Autodesk Inventor part; units mm, degrees
ref_plane "YZ Plane" through (0, 0, 0) normal (1, 0, 0) x (0, 1, 0)
ref_plane "XZ Plane" through (0, 0, 0) normal (0, 1, 0) x (-1, 0, 0)
ref_plane "XY Plane" through (0, 0, 0) normal (0, 0, 1) x (1, 0, 0)
sketch "Sketch1" plane through (0, 0, 0) normal (0, 0, 1) x (1, 0, 0)
  circle A0 centre (0, 0) radius 22.4676
  circle A1 centre (0, 0) radius 6.35
  point P0 (0, 17.5006)
  point P1 (-17.5006, 0)
  point P2 (0, -17.5006)
  point P3 (17.5006, 0)
  dimension "d0" = 44.9351
  dimension "d1" = 12.7
  dimension "d6" = 35.0012
  dimension "d7" = 17.5006
  dimension "d8" = 17.5006
  dimension "d9" = 17.5006
  dimension "d10" = 17.5006
extrude "Extrusion1" add sketch "Sketch1" along normal blind 132.715 contours A0 | A1
extrude "Extrusion2" add sketch "Sketch1" against normal blind 23.5128 contours A1
hole "Hole1" at (0, 17.5006, 0) at (-17.5006, 0, 0) at (0, -17.5006, 0) at (17.5006, 0, 0) direction (0, 0, 1) diameter 3.5052 end through all
thread "Thread1"
thread "Thread2"
thread "Thread3"
thread "Thread4"
The listing builds one solid part. Answer for the finished solid, in the listing's coordinates (mm). Coordinates: 2 decimals unless noted, no trailing zeros. Loops run counter-clockwise (first coordinate to the right, second up) from the corner with the lowest first, then second, coordinate; pieces in that order, holes last. Notation, with made-up numbers: M -26.75,43 L -5.75,43 A35 ccw -5.75,76 Z; hole C 21.5,-17 d2. An arc over 180 degrees is marked long. Answer as a JSON object with one key per item and string values. Group by question number.
Item 1: Section A-A (y = 0) is taken. Write down the section's boundary in (x, z) (3 decimals).
Item 2: Determine the mould class of faces 1 (the face through (-0.53, -15.83, 67.29)), 2 (the face through (-1.38, -6.2, -11.59)), 3 (the face through (5, -5, 0)) for opening direction Y: +Y half, -Y half, draft (parallel to the pull), parting line (faces both ways), or undercut.
Item 3: Section D-D (z = 112) is taken. Write down the section's boundary in (x, y).
Item 4: Consider L1, parallel to Y at x = 0, z = 94.5; L2, parallel to Y at x = -17, z = 11.5; L3, parallel to Z at x = -6, y = 20 (3 decimals). Determine where each line is inside the solid, lowest interval first.
Item 5: Section C-C (y = -17.5) is taken. Write down the section's boundary in (x, z) (3 decimals).
Item 6: Each of these flat-tipped pins is pushed along its axis until it touches: P1, Ø1.5, axis at x = -12, y = 8, coming from the -Z side; P2, Ø5, axis at x = -15.5, z = 60, coming from the -Y side; P3, Ø2, axis at x = 7.5, z = 105.5, coming from the -Y side. Where does it stop, or does it pass through?
Solved:
{
 "1": {"outline": "M -22.468,0 L -19.253,0 L -19.253,132.715 L -22.468,132.715 Z; M -15.748,0 L -6.35,0 L -6.35,-23.513 L 6.35,-23.513 L 6.35,0 L 15.748,0 L 15.748,132.715 L -15.748,132.715 Z; M 19.253,0 L 22.468,0 L 22.468,132.715 L 19.253,132.715 Z"},
 "2": {"face 1": "undercut", "face 2": "parting line", "face 3": "draft"},
 "3": {"outline": "C 0,0 d44.94; hole C -17.5,0 d3.51; hole C 0,-17.5 d3.51; hole C 0,17.5 d3.51; hole C 17.5,0 d3.51"},
 "4": {"L1": "y = -22.47 to -19.25, -15.75 to 15.75, 19.25 to 22.47", "L2": "y = -14.69 to -1.68, 1.68 to 14.69", "L3": "z = 0 to 132.715"},
 "5": {"outline": "M -14.091,0 L -1.753,0 L -1.753,132.715 L -14.091,132.715 Z; M 1.753,0 L 14.091,0 L 14.091,132.715 L 1.753,132.715 Z"},
 "6": {"P1": "stops at z = 0", "P2": "stops at y = -18.32", "P3": "stops at y = -21.51"}
}
